Geometry: final body of the model. Coordinates: model frame, mm. A direction names the side the tool comes from. Coordinates: 2 decimals unless noted, no trailing zeros. Loops run counter-clockwise (first coordinate to the right, second up) from the corner with the lowest first, then second, coordinate; pieces in that order, holes last. Notation, with made-up numbers: (2, 21) - (58, 21) arc R21 ccw to (58, 49) - close; hole circle Ø9 at (-7, 85). An arc over 180 degrees is marked (long way). Put each result on its own line as item: value. Start each with the question number.
1) Contact query for flat-ended pins moving along their axis: pin 1 Ø9 at (y, z) = (10, 81) entering from +X; pin 2 Ø1 at (y, z) = (11, 78) entering from -X; pin 3 Ø3 at (y, z) = (9, 59) entering from -X; pin 4 Ø5 at (x, z) = (28.55, 5.22) entering from +Y (1 decimal). Output: stop coordinate, or through.
2) Section A-A on z = 73. Output: boundary loops of the cut face in (x, y), and give its area (3 significant figures).
3) Material intervals for line 1 along X through (y, z) = (4.5, 75.5); line 2 along X through (y, z) = (9.5, 24.5); line 3 along X through (y, z) = (7.5, 7.5), sorted ascending. Write a range as from..to.
4) Section D-D on z = 13. Output: boundary loops of the cut face in (x, y).
5) Section C-C on x = -9. Output: boundary loops of the cut face in (y, z).
6) Draft query along Z for faces 4 (the flat face through (50.19, 8.87, 39.46)), 5 (the flat face through (-2, 18, 5)), 6 (the flat face through (1, 9, -11.726)), 7 (the cylindrical face through (-1.718, 8.874, 14.797)). Return one class per face: +Z half, -Z half, draft (parallel to the pull), parting line (faces both ways), or undercut.
7) Section B-B on y = 12. Output: boundary loops of the cut face in (x, z), and give its area (3 significant figures).
8) Reachability of faces 1 (the flat face through (-2.625, 9, 78)), 2 (the flat face through (-20.625, 9, 80)), 3 (the flat face through (19.375, 9, 80)) from +Z, -Z, +X, -X, +Y, -Y: full face, straight path, thin tool, end or side. Return the list, or none.
```python
from build123d import *

# Parameters (mm, degrees)
EXTRUDE1_DEPTH           = 18
F_6_0_6_DIAMETER_HOLE1_D = 6


with BuildPart() as part:
    # Sketch1 → Extrude1 (new body)
    with BuildSketch(Plane(origin=(0, 0, 0), x_dir=(1, 0, 0), z_dir=(0, 1, 0))):
        with BuildLine():
            Line((-83.124824855, -7.773679355), (-20.624824855, -70.273679355))
            Line((-20.624824855, -70.273679355), (-20.624824855, -90.273679355))
            Line((-20.624824855, -90.273679355), (-2.624824855, -90.273679355))
            Line((-2.624824855, -90.273679355), (-2.624824855, -65.695126993))
            ThreePointArc((-2.624824855, -65.695126993), (-0.624824855, -14.773679355), (1.375175145, -65.695126993))
            Line((1.375175145, -65.695126993), (1.375175145, -90.273679355))
            Line((1.375175145, -90.273679355), (19.375175145, -90.273679355))
            Line((19.375175145, -90.273679355), (19.375175145, -70.273679355))
            Line((19.375175145, -70.273679355), (81.875175145, -7.773679355))
            Line((81.875175145, -7.773679355), (81.875175145, 11.726320645))
            Line((81.875175145, 11.726320645), (-83.124824855, 11.726320645))
            Line((-83.124824855, 11.726320645), (-83.124824855, -7.773679355))
        make_face()
    extrude(amount=EXTRUDE1_DEPTH)

    # Ø6.0 (6) Diameter Hole1 (through all)
    with Locations(Plane(origin=(-34.816928484, 18, 5.785627569), x_dir=(0, 0, 1), z_dir=(0, 1, 0))):
        with Locations((0, 0), (-0.569202013, 63.371157488)):
            Hole(F_6_0_6_DIAMETER_HOLE1_D / 2)


solid = part.part
```
Answer block:
1. pin 1: stops at x = 19.38
1. pin 2: stops at x = -20.62
1. pin 3: stops at x = -33.4
1. pin 4: passes through
2. outline: (-20.62, 0) - (-2.62, 0) - (-2.62, 18) - (-20.62, 18) - close; (1.38, 0) - (19.38, 0) - (19.38, 18) - (1.38, 18) - close
2. area: 648 mm²
3. line 1: x = -20.62..-2.62, 1.38..19.38
3. line 2: x = -66.4..-20.66, 19.41..65.15
3. line 3: x = -83.12..-37.28, -32.36..26.61, 30.5..81.88
4. outline: (-77.9, 0) - (76.65, 0) - (76.65, 18) - (-77.9, 18) - close
5. outline: (0, -11.73) - (18, -11.73) - (18, 16.19) - (0, 16.19) - close; (0, 64.36) - (18, 64.36) - (18, 90.27) - (0, 90.27) - close
6. face 4: +Z half
6. face 5: draft
6. face 6: -Z half
6. face 7: undercut
7. outline: (-83.12, -11.73) - (81.88, -11.73) - (81.88, 7.77) - (19.38, 70.27) - (19.38, 90.27) - (1.38, 90.27) - (1.38, 65.7) arc R25.5 cw (long way) to (-2.62, 65.7) - (-2.62, 90.27) - (-20.62, 90.27) - (-20.62, 70.27) - (-83.12, 7.77) - close; hole circle Ø6 at (-34.82, 5.79); hole circle Ø6 at (28.55, 5.22)
7. area: 8,230 mm²
8. face 1: +Z, +Y, -Y
8. face 2: +Z, -X, +Y, -Y
8. face 3: +Z, +X, +Y, -Y
